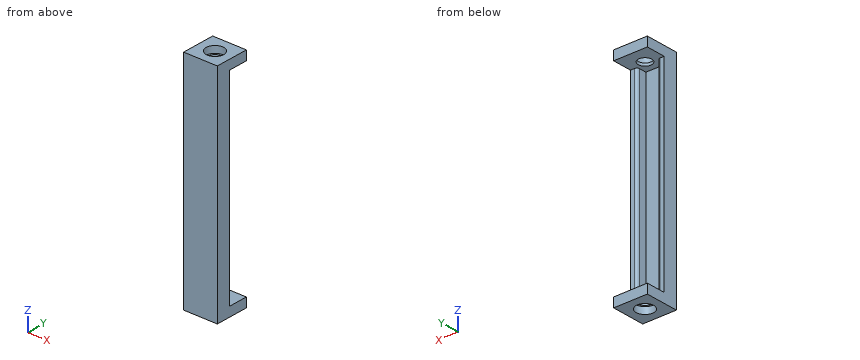
Autodesk Inventor part; units mm, degrees
ref_plane "YZ Plane" through (0, 0, 0) normal (1, 0, 0) x (0, 1, 0)
ref_plane "XZ Plane" through (0, 0, 0) normal (0, 1, 0) x (-1, 0, 0)
ref_plane "XY Plane" through (0, 0, 0) normal (0, 0, 1) x (1, 0, 0)
sketch "Sketch1" plane through (0, 0, 0) normal (0, 1, 0) x (-1, 0, 0)
  line L0 (0, 0) -> (25, 0)
  line L1 (25, 0) -> (25, -165)
  line L2 (25, -165) -> (0, -165)
  line L3 (0, -165) -> (0, 0)
  dimension "d0" = 25
  dimension "d1" = 165
extrude "Extrusion1" add sketch "Sketch1" along normal blind 3
sketch "Sketch2" plane through (0, 3, 0) normal (0, 1, 0) x (1, 0, 0)
  line L0 (-25, 165) -> (-25, 0)
  line L1 (0, 0) -> (0, 165)
  line L2 (-25, 0) -> (0, 0)
  line L3 (0, 0) -> (0, 7)
  line L4 (0, 7) -> (-25, 7)
  line L5 (-25, 7) -> (-25, 0)
  line L6 (0, 165) -> (-25, 165)
  line L7 (-25, 165) -> (0, 165)
  line L8 (0, 165) -> (0, 158)
  line L9 (0, 158) -> (-25, 158)
  line L10 (-25, 158) -> (-25, 165)
  dimension "d4" = 7
  dimension "d5" = 7
extrude "Extrusion2" add sketch "Sketch2" along normal blind 22 contours L6 L1 L9 L0 | L4 L1 L2 L0
sketch "Sketch3" plane through (-25, 0, 0) normal (0, 0, 1) x (1, 0, 0)
  point P0 (25, 0)
sketch "Sketch4" plane through (-25, 0, 0) normal (0, 0, 1) x (1, 0, 0)
  line L0 (25, 25) -> (0, 25) construction
  line L1 (25, 0) -> (0, 25) construction
  circle A0 centre (12.5, 12.5) radius 6.5
  dimension "d8" = 13
extrude "Extrusion3" cut sketch "Sketch4" against normal blind 5
sketch "Sketch5" plane through (0, 0, -165) normal (0, 0, -1) x (-1, 0, 0)
  circle A0 centre (12.5, 12.5) radius 6.5
  circle A1 centre (12.5, 12.5) radius 6.5
  point P0 (0, 0)
extrude "Extrusion4" cut sketch "Sketch5" against normal blind 5
sketch "Sketch6" plane through (-25, 0, 0) normal (0, 0, 1) x (1, 0, 0)
  circle A0 centre (12.5, 12.5) radius 6.5
  circle A1 centre (12.5, 12.5) radius 5
  point P0 (25, 0)
  dimension "d13" = 10
extrude "Extrusion5" cut sketch "Sketch6" against normal blind 165 contours A1
sketch "Sketch7" plane through (-25, 3, -158) normal (0, 0, 1) x (1, 0, 0)
  line L0 (25, 0) -> (25, 22) construction
  line L1 (0, 0) -> (0, 22) construction
  point P0 (25, -3)
sketch "Sketch8" plane through (-25, 3, -158) normal (0, 0, 1) x (1, 0, 0)
  circle A0 centre (12.5, 9.5) radius 5
  point P0 (25, -3)
sketch "Sketch9" plane through (0, 3, 0) normal (0, 1, 0) x (1, 0, 0)
  line L0 (-25, 158) -> (0, 158)
  line L1 (0, 7) -> (-25, 7)
  line L2 (-25, 158) -> (-20, 158)
  line L3 (-20, 158) -> (-20, 7)
  line L4 (-20, 7) -> (-25, 7)
  line L5 (-25, 7) -> (-25, 158)
  line L6 (0, 0) -> (0, 7)
  line L7 (0, 7) -> (-5, 7)
  line L8 (-5, 7) -> (-5, 158)
  line L9 (-5, 158) -> (0, 158)
  line L10 (0, 158) -> (0, 7)
  dimension "d16" = 5
  dimension "d17" = 5
extrude "Extrusion6" add sketch "Sketch9" along normal blind 7.5 contours L0 L3 L1 L5 | L0 L10 L1 L8
fillet "Fillet1" radius 2 2 edges at (-5, 10.5, -82.5) (-20, 10.5, -82.5)
properties part number "baseAxel 11-28"
CAD build for the part. Positions are in the model's coordinates, mm. Round coordinates to 2 decimals unless told otherwise and drop trailing zeros. Loops run counter-clockwise (first coordinate to the right, second up) from the corner with the lowest first, then second, coordinate; pieces in that order, holes last. Notation, with made-up numbers: (-11, 33.5) - (41, 33.5) arc R14 cw to (41, 49.5) - close; hole circle Ø4 at (10.25, 84.25). An arc over 180 degrees is marked (long way). Return JSON: item names as keys, results as strings. Group by question number.
Q1. Drill centre lines: line 1 along Z through (x, y) = (-21.5, 21.75); line 2 along X through (y, z) = (8, -121); line 3 along Z through (x, y) = (-18, 12.75). Where is each one in solid material? Low to high. Write a range as [from, to].
Q2. Band-saw the part on C-C on z = -90. Give the cut face in (x, y), plus the area to 3 significant figures.
Q3. Flat gauge pins, fed straight in: pin 1 Ø6 at (x, y) = (-22.5, 18.5) entering from +Z; pin 2 Ø4 at (x, y) = (-15.5, 10) entering from -Z; pin 3 Ø2.5 at (x, z) = (-2, -50) entering from +Y; pin 4 Ø9 at (x, y) = (-12.5, 12.5) entering from -Z. Where does each tip first touch, or does it go through?
Q4. Band-saw the part on D-D on y = 15. Give the cut face in (x, z), plus the area to 3 significant figures.
Q5. Band-saw the part on B-B on y = 21. Give the cut face in (x, z), plus the area to 3 significant figures.
Q6. Band-saw the part on A-A on x = -12.5. Give the cut face in (y, z), plus the area to 3 significant figures.
Solutions:
{
 "1": {"line 1": "z = [-165, -158], [-7, 0]", "line 2": "x = [-25, -20], [-5, 0]", "line 3": "z = [-160, -158], [-7, -5]"},
 "2": {"outline": "(-25, 0) - (0, 0) - (0, 10.5) - (-3, 10.5) arc R2 ccw to (-5, 8.5) - (-5, 3) - (-20, 3) - (-20, 8.5) arc R2 ccw to (-22, 10.5) - (-25, 10.5) - close", "area": "148 mm^2"},
 "3": {"pin 1": "stops at z = 0", "pin 2": "stops at z = -160", "pin 3": "stops at y = 10.5", "pin 4": "passes through"},
 "4": {"outline": "(-25, -165) - (-18.5, -165) - (-18.5, -160) - (-16.83, -160) - (-16.83, -158) - (-25, -158) - close; (-25, -7) - (-16.83, -7) - (-16.83, -5) - (-18.5, -5) - (-18.5, 0) - (-25, 0) - close; (-8.17, -160) - (-6.5, -160) - (-6.5, -165) - (0, -165) - (0, -158) - (-8.17, -158) - close; (-8.17, -7) - (0, -7) - (0, 0) - (-6.5, 0) - (-6.5, -5) - (-8.17, -5) - close", "area": "195 mm^2"},
 "5": {"outline": "(-25, -165) - (0, -165) - (0, -158) - (-25, -158) - close; (-25, -7) - (0, -7) - (0, 0) - (-25, 0) - close", "area": "350 mm^2"},
 "6": {"outline": "(0, -165) - (6, -165) - (6, -160) - (7.5, -160) - (7.5, -158) - (3, -158) - (3, -7) - (7.5, -7) - (7.5, -5) - (6, -5) - (6, 0) - (0, 0) - close; (17.5, -160) - (19, -160) - (19, -165) - (25, -165) - (25, -158) - (17.5, -158) - close; (17.5, -7) - (25, -7) - (25, 0) - (19, 0) - (19, -5) - (17.5, -5) - close", "area": "633 mm^2"}
}
